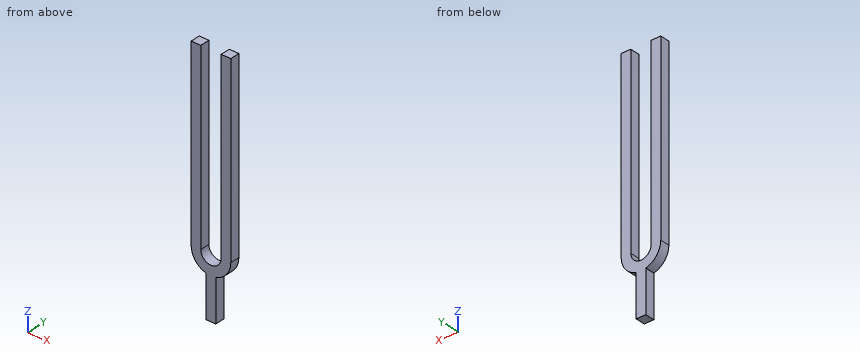
from build123d import *

# Parameters (mm, degrees)
F1_DEPTH = 1.9685
F3_W     = 3.937
F3_H     = 3.937


with BuildPart() as f1:
    # F0 (on Front) → F1 (new body, symmetric)
    with BuildSketch(Plane.XZ):
        with BuildLine():
            Line((-4.1529, 75.1713), (-8.0899, 75.1713))
            Line((-8.0899, 75.1713), (-8.0899, 0))
            ThreePointArc((-8.0899, 0), (0, -8.0899), (8.0899, 0))
            Line((8.0899, 0), (8.0899, 75.1713))
            Line((8.0899, 75.1713), (4.1529, 75.1713))
            Line((4.1529, 75.1713), (4.1529, 0))
            ThreePointArc((4.1529, 0), (0, -4.1529), (-4.1529, 0))
            Line((-4.1529, 0), (-4.1529, 75.1713))
        make_face()
    extrude(amount=F1_DEPTH, both=True)

    # F3 (on offset) → F4 (join, up to the next surface of F1)
    with BuildSketch(Plane.XY.offset(-25)):
        Rectangle(F3_W, F3_H)
    extrude(until=Until.NEXT)


solid = f1.part
Read the model definition and answer for the solid it produces. Units are mm, in the model's axes. Coordinates: 2 decimals unless noted, no trailing zeros. Loops run counter-clockwise (first coordinate to the right, second up) from the corner with the lowest first, then second, coordinate; pieces in that order, holes last. Notation, with made-up numbers: (37, 25) -> (96, 25) arc R10 ccw to (96, 36) -> close; hole circle Ø6 at (45.25, 83.5). An arc over 180 degrees is marked (long way). Write item = value, one per line. Start each with the question number.
1) Given P1, Ø1, axis at y = 1.5, z = -7, coming from the -X side; P2, Ø1, axis at x = 2.5, y = -1.5, coming from the -Z side; P3, Ø1.2, axis at y = 0.5, z = -20, coming from the -X side, each flat-ended and moving along its own axis, determine where each tip first touches the part or whether it passes through.
2) Find the intervals of material crossed by L1, parallel to X at y = -0.5, z = 23; L2, parallel to X at y = -0.5, z = -13.5; L3, parallel to Z at x = 2.5, y = -0.65, in increasing order. Write a range as from..to.
3) The part is cut by section C-C, the plane x = 0. Determine the outline of the cut face in (y, z), plus the area to 3 significant figures.
4) The part is cut by section B-B, the plane y = -1.2. Determine the outline of the cut face in (x, z).
5) The part is cut by section A-A, the plane z = 17.5. Determine the outline of the cut face in (x, y), plus the area to 3 significant figures.
6) The part is cut by section D-D, the plane x = -6.5. Determine the outline of the cut face in (y, z).
Result:
q1.P1 = -4.82
q1.P2 = -7.84
q1.P3 = -1.97
q2.L1 = -8.09..-4.15, 4.15..8.09
q2.L2 = -1.97..1.97
q2.L3 = -7.69..-3.32
q3.outline = (-1.97, -25) -> (1.97, -25) -> (1.97, -4.15) -> (-1.97, -4.15) -> close
q3.area = 82.1 mm²
q4.outline = (-8.09, 0) arc R8.09 ccw to (-1.97, -7.85) -> (-1.97, -25) -> (1.97, -25) -> (1.97, -7.85) arc R8.09 ccw to (8.09, 0) -> (8.09, 75.17) -> (4.15, 75.17) -> (4.15, 0) arc R4.15 cw to (-4.15, 0) -> (-4.15, 75.17) -> (-8.09, 75.17) -> close
q5.outline = (-8.09, -1.97) -> (-4.15, -1.97) -> (-4.15, 1.97) -> (-8.09, 1.97) -> close; (4.15, -1.97) -> (8.09, -1.97) -> (8.09, 1.97) -> (4.15, 1.97) -> close
q5.area = 31.0 mm²
q6.outline = (-1.97, -4.82) -> (1.97, -4.82) -> (1.97, 75.17) -> (-1.97, 75.17) -> close
